Here's how the part is built. I have some questions about the finished solid (model axes, mm). Give positions to 0.01 mm unless a question says otherwise; leave off trailing zeros. Loops run counter-clockwise (first coordinate to the right, second up) from the corner with the lowest first, then second, coordinate; pieces in that order, holes last. Notation, with made-up numbers: M 85,67 L 113,67 A31 cw 113,104 Z; hole C 56,87 d10. An arc over 180 degrees is marked long. Answer as CSV lines item,"result". Start each with the question number.
Item 1: I want a section at A-A on z = -37.5. List the corners of the cut face in (x, y) for me.
Item 2: I want a section at D-D on y = 4.05. Give the number of separate pieces and of enclosed holes in the cut face, plus the area to 3 significant figures.
Item 3: I want a section at B-B on x = -15.5. List the corners of the cut face in (y, z) for me, plus the area to 3 significant figures.
Item 4: I want a section at C-C on z = 18.5. List the corners of the cut face in (x, y) for me, plus the area to 3 significant figures.
Item 5: If I drill on line 1 along Z through (x, y) = (-15.5, 1.1); line 2 along X through (y, z) = (3.35, -6.5); line 3 along X through (y, z) = (3.45, 28.5), over which ranges is the centre line in solid material (lowest first)? Write a range as from..to.
Item 6: Will this pin go through, and if not, where does the flat tip stop? P1, Ø2.5, axis at x = -15.5, z = -37.5, coming from the -Y side.
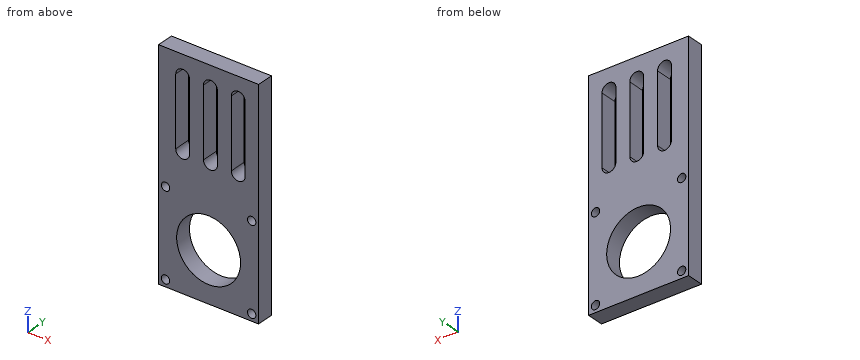
from build123d import *

# Parameters (mm, degrees)
SKETCH1_W           = 36
SKETCH1_H           = 80
SKETCH1_R           = 11.5
SKETCH1_R_2         = 1.5
BOSS_EXTRUDE1_DEPTH = 6


with BuildPart() as part:
    # Sketch1 → Boss-Extrude1 (new body)
    with BuildSketch(Plane(origin=(0, 0, 0), x_dir=(1, 0, 0), z_dir=(0, 1, 0))):
        Rectangle(SKETCH1_W, SKETCH1_H)
        with Locations((0, 22)):
            Circle(SKETCH1_R, mode=Mode.SUBTRACT)
        with Locations((-15.5, 37.5)):
            Circle(SKETCH1_R_2, mode=Mode.SUBTRACT)
        with Locations((15.5, 37.5)):
            Circle(SKETCH1_R_2, mode=Mode.SUBTRACT)
        with Locations((15.5, 6.5)):
            Circle(SKETCH1_R_2, mode=Mode.SUBTRACT)
        with Locations((-15.5, 6.5)):
            Circle(SKETCH1_R_2, mode=Mode.SUBTRACT)
        with BuildLine():
            Line((-1.827248673, -32.5), (-1.827248673, -7.5))
            ThreePointArc((-1.827248673, -7.5), (0.672751327, -5), (3.172751327, -7.5))
            Line((3.172751327, -7.5), (3.172751327, -32.5))
            ThreePointArc((3.172751327, -32.5), (0.672751327, -35), (-1.827248673, -32.5))
        make_face(mode=Mode.SUBTRACT)
        with BuildLine():
            Line((8.172751327, -32.5), (8.172751327, -7.5))
            ThreePointArc((8.172751327, -7.5), (10.672751327, -5), (13.172751327, -7.5))
            Line((13.172751327, -7.5), (13.172751327, -32.5))
            ThreePointArc((13.172751327, -32.5), (10.672751327, -35), (8.172751327, -32.5))
        make_face(mode=Mode.SUBTRACT)
        with BuildLine():
            Line((-6.827248673, -32.5), (-6.827248673, -7.5))
            ThreePointArc((-6.827248673, -7.5), (-9.327248673, -5), (-11.827248673, -7.5))
            Line((-11.827248673, -7.5), (-11.827248673, -32.5))
            ThreePointArc((-11.827248673, -32.5), (-9.327248673, -35), (-6.827248673, -32.5))
        make_face(mode=Mode.SUBTRACT)
    extrude(amount=BOSS_EXTRUDE1_DEPTH)


solid = part.part
Result:
1,outline,"M -18,0 L -17,0 L -17,6 L -18,6 Z; M -14,0 L 14,0 L 14,6 L -14,6 Z; M 17,0 L 18,0 L 18,6 L 17,6 Z"
2,separate pieces,"1"
2,enclosed holes,"8"
2,area,"2,000 mm^2"
3,outline,"M 0,-40 L 6,-40 L 6,-39 L 0,-39 Z; M 0,-36 L 6,-36 L 6,-8 L 0,-8 Z; M 0,-5 L 6,-5 L 6,40 L 0,40 Z"
3,area,"444 mm^2"
4,outline,"M -18,0 L -11.83,0 L -11.83,6 L -18,6 Z; M -6.83,0 L -1.83,0 L -1.83,6 L -6.83,6 Z; M 3.17,0 L 8.17,0 L 8.17,6 L 3.17,6 Z; M 13.17,0 L 18,0 L 18,6 L 13.17,6 Z"
4,area,"126 mm^2"
5,line 1,"-40..-39, -36..-8, -5..40"
5,line 2,"-18..-17, -14..14, 17..18"
5,line 3,"-18..-11.83, -6.83..-1.83, 3.17..8.17, 13.17..18"
6,P1,"through"
